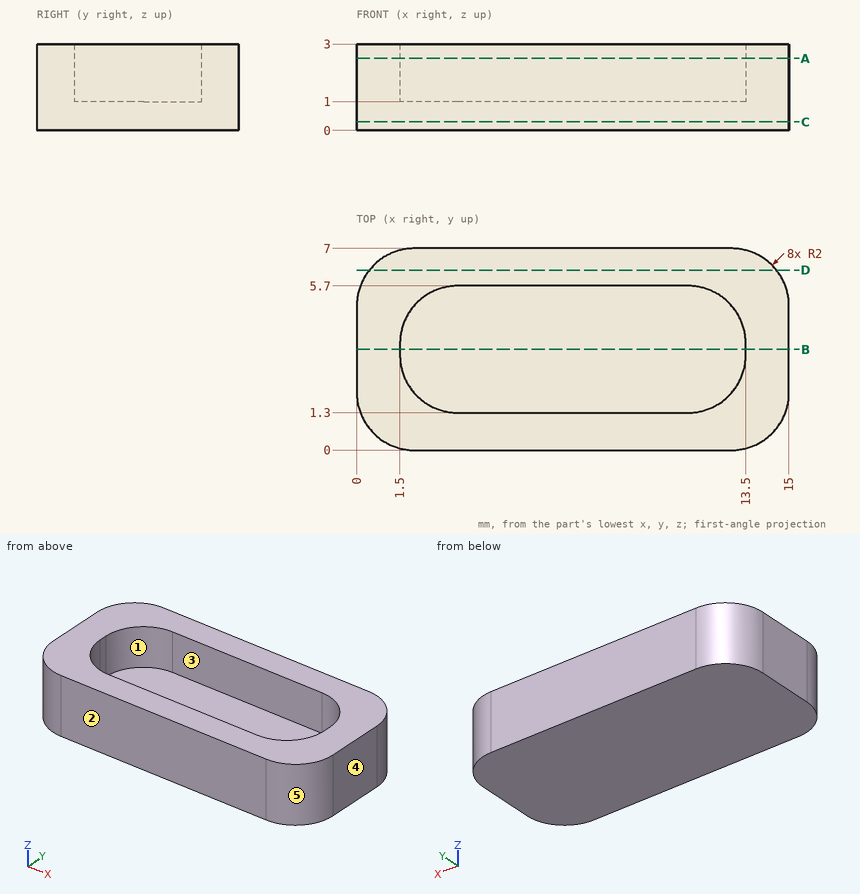
Here's the drawing with two shaded views (mm, measured from the low corner). I have some questions. A direction names the side the tool comes from. Give positions to 0.01 mm unless a question says otherwise; leave off trailing zeros. Loops run counter-clockwise (first coordinate to the right, second up) from the corner with the lowest first, then second, coordinate; pieces in that order, holes last. Notation, with made-up numbers: M 55.25,5.25 L 77.25,5.25 A7 cw 77.25,16.25 Z; hole C 12,86 d1. An arc over 180 degrees is marked long. Use one line per item in the form item = value. Start each with the question number.
(1) I want a section at D-D, the plane y = 6.25. Write out the boundary of the cut face in (x, z), and give its area (3 significant figures).
(2) I want a section at B-B, the plane y = 3.5. Write out the boundary of the cut face in (x, z), and give its area (3 significant figures).
(3) I'm going to push a flat-ended pin straight in: P1, Ø1.5, axis at x = 10.5, y = 4.5, coming from the +Z side. Where does the tip first touch, or does it pass through?
(4) I want a section at C-C, the plane z = 0.3. Write out the boundary of the cut face in (x, y).
(5) On a 3-axis mill with a long thin cutter (end or side, diameter ignored), from which of +Z, -Z, +X, -X, +Y, -Y can I reach the whole of each face in a straight line? I mean the marked faces 1 and 2. Say none if no direction works.
(6) Please list where these lines run through material, in increasing order: line 1 (Y direction, x = 4.25, z = 1.2); line 2 (Y direction, x = 12.5, z = 2.05); line 3 (Z direction, x = 12.25, y = 4).
(7) Thinking about a two-plate mould opening in Y: for the marked faces 3, 4 and 5, which applies, released by +Y, released by -Y, zero draft, split by the parting line, or undercut?
(8) I want a section at A-A, the plane z = 2.5. Write out the boundary of the cut face in (x, y).
Worked out:
q1.outline = M 0.44,0 L 14.56,0 L 14.56,3 L 0.44,3 Z
q1.area = 42.4 mm²
q2.outline = M 0,0 L 15,0 L 15,3 L 13.5,3 L 13.5,1 L 1.5,1 L 1.5,3 L 0,3 Z
q2.area = 21.0 mm²
q3.P1 = 1
q4.outline = M 0,2 A2 ccw 2,0 L 13,0 A2 ccw 15,2 L 15,5 A2 ccw 13,7 L 2,7 A2 ccw 0,5 Z
q5.face_1 = +Z
q5.face_2 = +Z, -Z, +X, -X, -Y
q6.line_1 = 0 to 1.3, 5.7 to 7
q6.line_2 = 0 to 1.57, 5.43 to 7
q6.line_3 = 0 to 1
q7.face_3 = undercut
q7.face_4 = zero draft
q7.face_5 = released by -Y
q8.outline = M 0,2 A2 ccw 2,0 L 13,0 A2 ccw 15,2 L 15,5 A2 ccw 13,7 L 2,7 A2 ccw 0,5 Z; hole M 1.5,3.3 A2 ccw 3.5,1.3 L 11.5,1.3 A2 ccw 13.5,3.3 L 13.5,3.7 A2 ccw 11.5,5.7 L 3.5,5.7 A2 ccw 1.5,3.7 Z
